Autodesk Inventor part; units mm, degrees
ref_plane "YZ Plane" through (0, 0, 0) normal (1, 0, 0) x (0, 1, 0)
ref_plane "XZ Plane" through (0, 0, 0) normal (0, 1, 0) x (-1, 0, 0)
ref_plane "XY Plane" through (0, 0, 0) normal (0, 0, 1) x (1, 0, 0)
sketch "スケッチ1" plane through (0, 0, 0) normal (1, 0, 0) x (0, 1, 0)
  circle A0 centre (0, 0) radius 6
  circle A1 centre (5, -30) radius 11
  line L0 (-6, 0) -> (-6, -30)
  line L1 (5.6757, 1.9459) -> (15.4054, -26.4324)
  circle A2 centre (5, -30) radius 12.5
  circle A3 centre (0, 0) radius 3
  circle A4 centre (5, -30) radius 1.75
  line L2 (5, -30) -> (5, -41) construction
  circle A5 centre (0, 0) radius 4.5 construction
  circle A6 centre (5, -30) radius 2.5 construction
  line L3 (4.4778, 0.4463) -> (7.4877, -29.7521) construction
  line L4 (2.5664, -30.5723) -> (-4.3805, -1.0301) construction
  circle A7 centre (2.3696, -14.2177) radius 2
  circle A8 centre (2.3696, -14.2177) radius 1
  circle A9 centre (2.3696, -14.2177) radius 3.5522 construction
  line L5 (9.4297, -56.5784) -> (-3.4387, 20.6324) construction
  circle A10 centre (5, -30) radius 14 construction
  point P0 (-6, -24.0628)
  point P1 (13.4798, -20.8162)
  point P2 (15.9919, -30.4228)
  point P3 (-1.7415, -38.692)
  point P4 (13.8604, -21.1828)
  point P5 (-6.4987, -25.098)
  dimension "d0" = 12
  dimension "d1" = 22
  dimension "d2" = 30
  dimension "d3" = 25
  dimension "d4" = 6
  dimension "d5" = 3.5
  dimension "d21" = 9
  dimension "d22" = 5
  dimension "d23" = 2
  dimension "d24" = 4
  dimension "d35" = 28
extrude "押し出し1" add sketch "スケッチ1" against normal blind 2.5 contours A0 | A0 L1 A2 L0 | A2 L0 A1 L1 | L1 A1 L0 A2 | A1 | A3 | A7 | A8
sketch "スケッチ2" plane through (-2.5, 0, 0) normal (-1, 0, 0) x (0, 0, 1)
  circle A0 centre (0, 0) radius 3.6
  circle A1 centre (0, 0) radius 3
  dimension "d8" = 7.2
extrude "押し出し2" cut sketch "スケッチ2" against normal blind 0.6
hole "穴1" at (0, 2.3696, -14.2177) direction (-1, 0, 0) diameter 3.2 end through all counterbore diameter 4 counterbore depth 1
hole "穴2" at (0, 0, 0) direction (-1, 0, 0) diameter 6 end through all counterbore diameter 7.5 counterbore depth 0.6
properties part number "Main_Frame"
CAD build for the part. Positions are in the model's coordinates, mm. A direction names the side the tool comes from. Round coordinates to 2 decimals unless told otherwise and drop trailing zeros. Loops run counter-clockwise (first coordinate to the right, second up) from the corner with the lowest first, then second, coordinate; pieces in that order, holes last.
(1) Two-plate mould, pull along Y, no slides. Class faces 1 (the cylindrical face through (-1.232, 6.669, -42.388)), 2 (the flat face through (-2.5, 5, -23)), 3 (the cylindrical face through (-1.23, 3.61, -31.06)), 4 (the flat face through (-1.232, 9.523, -9.276)): +Y half, -Y half, draft (parallel to the pull), parting line (faces both ways), or undercut.
(2) Which spindle directions (+Z, -Z, +X, -X, +Y, -Y) get a long thin tool onto all of the face, cutting with end or side? Do faces 5 (the flat face through (-1, 1, -13)), 6 (the cylindrical face through (-2.204, 1.081, 3.434)), 7 (the cylindrical face through (-1, 0, 3)), 8 (the flat face through (-1, -6, -12)). Say none if no direction does.
(3) Cut at B-B (y = 5). Give the cut face in (x, z).
(4) Cut at D-D (z = -15). Give the cut face in (x, y), plus the area to 3 significant figures.
(5) Cut at A-A (z = -30). Give the cut face in (x, y).
(6) Wall check: line 1 along Z through (x, y) = (-0.45, 1); line 2 along Z through (x, y) = (-1.6, 2); line 3 along Y through (x, z) = (-2.1, 0). Give the ranges that are in metal, low to high.
(7) Drop flat-ended pins along their axis: pin 1 (12 mm diameter, centred on y = 0.5, z = -13, fed in from +X); pin 2 (1.2 mm diameter, centred on x = -1, z = -18, fed in from -Y); pin 3 (2 mm diameter, centred on y = 5, z = -30, fed in from -X); pin 4 (1 mm diameter, centred on x = -2, z = -28, fed in from +Y). Give the stop position or say it passes through.
(8) Cut at C-C (x = -1.5). Give the cut face in (y, z).
Findings below:
1. face 1: parting line
1. face 2: draft
1. face 3: undercut
1. face 4: +Y half
2. face 5: +X
2. face 6: -X
2. face 7: +X, -X
2. face 8: +Z, +X, -X, -Y
3. outline: (-2.5, -42.5) - (0, -42.5) - (0, -31.75) - (-2.5, -31.75) - close; (-2.5, -28.25) - (0, -28.25) - (0, 3.32) - (-2.5, 3.32) - close
4. outline: (-2.5, -6) - (0, -6) - (0, 0.53) - (-1, 0.53) - (-1, 0.97) - (-2.5, 0.97) - close; (-2.5, 3.77) - (-1, 3.77) - (-1, 4.21) - (0, 4.21) - (0, 11.49) - (-2.5, 11.49) - close
4. area: 35.8 mm2
5. outline: (-2.5, -7.5) - (0, -7.5) - (0, 3.25) - (-2.5, 3.25) - close; (-2.5, 6.75) - (0, 6.75) - (0, 17.5) - (-2.5, 17.5) - close
6. line 1: z = -41.84 to -15.68, -12.76 to -3.61, 3.61 to 5.92
6. line 2: z = -42.13 to -15.77, -12.66 to -2.24, 2.24 to 5.66
6. line 3: y = -6 to -3.6, 3.6 to 6.34
7. pin 1: stops at x = 0
7. pin 2: stops at y = -6
7. pin 3: passes through
7. pin 4: stops at y = 17.41
8. outline: (-6, -24.06) arc R12.5 ccw (long way) to (13.48, -20.82) - (5.68, 1.95) arc R6 ccw to (-6, 0) - close; hole circle Ø6 at (0, 0); hole circle Ø3.2 at (2.37, -14.22); hole circle Ø3.5 at (5, -30)
